Geometry check sheet. Reference: drawing and pictorial views, mm from the part's lowest x, y, z. A direction names the side the tool comes from. Round coordinates to 2 decimals unless told otherwise and drop trailing zeros. Write each loop counter-clockwise with the first axis right and the second up, starting at its lowest first coordinate (ties: lowest second). Pieces come first, ordered by that corner, then holes. Notation, with made-up numbers: (64, 17.5) -> (97, 17.5) arc R18 cw to (97, 26.5) -> close; hole circle Ø4 at (53.25, 25). An arc over 180 degrees is marked (long way). Write item = value, one per line.
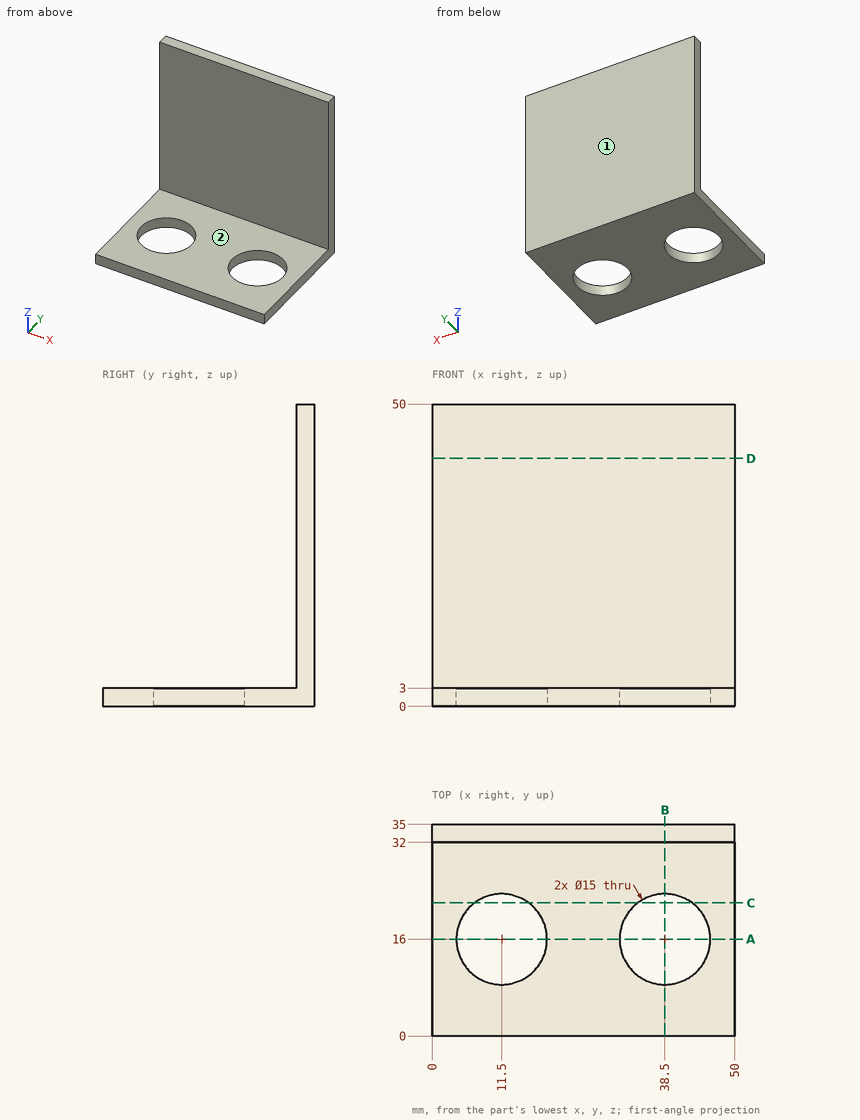
(1) Sectioned sample at A-A on y = 16. Enter the section's corners in (x, z).
Worked answers:
outline = (0, 0) -> (4, 0) -> (4, 3) -> (0, 3) -> close; (19, 0) -> (31, 0) -> (31, 3) -> (19, 3) -> close; (46, 0) -> (50, 0) -> (50, 3) -> (46, 3) -> close
(2) Sectioned sample at C-C on y = 22. Enter the section's corners in (x, z).
Worked answers:
outline = (0, 0) -> (7, 0) -> (7, 3) -> (0, 3) -> close; (16, 0) -> (34, 0) -> (34, 3) -> (16, 3) -> close; (43, 0) -> (50, 0) -> (50, 3) -> (43, 3) -> close
(3) Material ranges on L1, parallel to Y at x = 38.5, z = 1.5; L2, parallel to Y at x = 8, z = 11; L3, parallel to Z at x = 19, y = 2, recorded low to high. Write a range as [from, to].
Worked answers:
L1 = [0, 8.5], [23.5, 35]
L2 = [32, 35]
L3 = [0, 3]
(4) Sectioned sample at D-D on z = 41. Enter the section's corners in (x, y), then the cut area to 3 significant figures.
Worked answers:
outline = (0, 32) -> (50, 32) -> (50, 35) -> (0, 35) -> close
area = 150 mm²
(5) Access from +Z, -Z, +X, -X, +Y, -Y to the whole of each face (thin tool, end or side, straight path). Record for the marked faces 1 and 2.
Worked answers:
face_1 = +Z, -Z, +X, -X, +Y
face_2 = +Z, +X, -X, -Y
(6) Sectioned sample at B-B on x = 38.5. Enter the section's corners in (y, z).
Worked answers:
outline = (0, 0) -> (8.5, 0) -> (8.5, 3) -> (0, 3) -> close; (23.5, 0) -> (35, 0) -> (35, 50) -> (32, 50) -> (32, 3) -> (23.5, 3) -> close
(7) Go/stop test with flat-tipped pins: P1, Ø6, axis at x = 45, y = 4, coming from the +Z side; P2, Ø1.5, axis at x = 23.5, z = 21.5, coming from the -Y side. Record where each tip stops, or that it passes through.
Worked answers:
P1 = 3
P2 = 32
